Geometry check sheet. Reference: the model listing, model coordinates, mm. Coordinates: 2 decimals unless noted, no trailing zeros. Write each loop counter-clockwise with the first axis right and the second up, starting at its lowest first coordinate (ties: lowest second). Pieces come first, ordered by that corner, then holes. Notation, with made-up numbers: M 70.5,-33.5 L 120.5,-33.5 A23 cw 120.5,2.5 Z; hole C -8,40.25 d1. An arc over 180 degrees is marked long. Write item = value, one per line. Start each with the question number.
```python
from build123d import *

# Parameters (mm, degrees)
SKETCH5_W           = 40
SKETCH5_H           = 40
BOSS_EXTRUDE2_DEPTH = 2
CUT_EXTRUDE1_DEPTH  = 2
CUT_EXTRUDE4_DEPTH  = 2
CUT_EXTRUDE5_DEPTH  = 2
CUT_EXTRUDE6_DEPTH  = 2
CUT_EXTRUDE7_DEPTH  = 2
CUT_EXTRUDE8_DEPTH  = 2


with BuildPart() as part:
    # Sketch5 → Boss-Extrude2 (new body)
    with BuildSketch(Plane.XY):
        Rectangle(SKETCH5_W, SKETCH5_H)
    extrude(amount=BOSS_EXTRUDE2_DEPTH)

    # Sketch4 → Cut-Extrude1 (cut)
    with BuildSketch(Plane.XY):
        Polygon((18, 16.585786438), (18, 10.414213562), (14.914213562, 13.5), align=None)
        Polygon((10.414213562, 18.056847711), (16.585786438, 18.056847711), (13.5, 14.971061274), align=None)
    extrude(amount=CUT_EXTRUDE1_DEPTH, mode=Mode.SUBTRACT)

    # Sketch4_5 → Cut-Extrude4 (cut)
    with BuildSketch(Plane.XY):
        Polygon((-13.5, -14.914213562), (-16.585786438, -18), (-10.414213562, -18), align=None)
        Polygon((-5.914213562, -13.5), (-9, -16.585786438), (-12.085786438, -13.5), (-9, -10.414213562), align=None)
        Polygon((-13.5, -5.914213562), (-10.414213562, -9), (-13.5, -12.085786438), (-16.585786438, -9), align=None)
        Polygon((-18, -16.585786438), (-18, -10.414213562), (-14.914213562, -13.5), align=None)
    extrude(amount=CUT_EXTRUDE4_DEPTH, mode=Mode.SUBTRACT)

    # Sketch4_6 → Cut-Extrude5 (cut)
    with BuildSketch(Plane.XY):
        Polygon((-1.414213562, -18), (-7.585786438, -18), (-4.5, -14.914213562), align=None)
        Polygon((3.085786438, -13.5), (0, -16.585786438), (-3.085786438, -13.5), (0, -10.414213562), align=None)
        Polygon((7.585786438, -18), (1.414213562, -18), (4.5, -14.914213562), align=None)
        Polygon((12.085786438, -13.5), (9, -16.585786438), (5.914213562, -13.5), (9, -10.414213562), align=None)
        Polygon((13.5, -14.914213562), (16.585786438, -18), (10.414213562, -18), align=None)
        Polygon((18, -10.414213562), (18, -16.585786438), (14.914213562, -13.5), align=None)
        Polygon((13.5, -5.914213562), (16.585786438, -9), (13.5, -12.085786438), (10.414213562, -9), align=None)
        Polygon((4.5, -5.914213562), (7.585786438, -9), (4.5, -12.085786438), (1.414213562, -9), align=None)
        Polygon((12.085786438, -4.5), (9, -7.585786438), (5.914213562, -4.5), (9, -1.414213562), align=None)
        Polygon((18, -1.414213562), (18, -7.585786438), (14.914213562, -4.5), align=None)
    extrude(amount=CUT_EXTRUDE5_DEPTH, mode=Mode.SUBTRACT)

    # Sketch4_7 → Cut-Extrude6 (cut)
    with BuildSketch(Plane.XY):
        Polygon((13.5, 3.085786438), (16.585786438, 0), (13.5, -3.085786438), (10.414213562, 0), align=None)
        Polygon((18, 7.585786438), (18, 1.414213562), (14.914213562, 4.5), align=None)
        Polygon((13.5, 12.085786438), (16.585786438, 9), (13.5, 5.914213562), (10.414213562, 9), align=None)
        Polygon((12.085786438, 4.5), (9, 1.414213562), (5.914213562, 4.5), (9, 7.585786438), align=None)
        Polygon((4.5, 12.085786438), (7.585786438, 9), (4.5, 5.914213562), (1.414213562, 9), align=None)
        Polygon((12.085786438, 13.5), (9, 10.414213562), (5.914213562, 13.5), (9, 16.585786438), align=None)
        Polygon((1.357365851, 18.056847711), (7.642634149, 18.056847711), (4.5, 14.914213562), align=None)
        Polygon((3.085786438, 13.5), (0, 10.414213562), (-3.085786438, 13.5), (0, 16.585786438), align=None)
        Polygon((3.085786438, 4.5), (0, 1.414213562), (-3.085786438, 4.5), (0, 7.585786438), align=None)
        Polygon((4.5, 3.085786438), (7.585786438, 0), (4.5, -3.085786438), (1.414213562, 0), align=None)
        Polygon((3.085786438, -4.5), (0, -7.585786438), (-3.085786438, -4.5), (0, -1.414213562), align=None)
        Polygon((-4.5, -5.914213562), (-1.414213562, -9), (-4.5, -12.085786438), (-7.585786438, -9), align=None)
    extrude(amount=CUT_EXTRUDE6_DEPTH, mode=Mode.SUBTRACT)

    # Sketch4_9 → Cut-Extrude7 (cut)
    with BuildSketch(Plane.XY):
        Polygon((-9, 1.414213562), (-12.085786438, 4.5), (-9, 7.585786438), (-5.914213562, 4.5), align=None)
        Polygon((-4.5, 3.085786438), (-1.414213562, 0), (-4.5, -3.085786438), (-7.585786438, 0), align=None)
        Polygon((-9, -7.585786438), (-12.085786438, -4.5), (-9, -1.414213562), (-5.914213562, -4.5), align=None)
        Polygon((-13.5, 3.085786438), (-10.414213562, 0), (-13.5, -3.085786438), (-16.585786438, 0), align=None)
        Polygon((-18, -7.585786438), (-18, -1.414213562), (-14.914213562, -4.5), align=None)
        Polygon((-18, 1.414213562), (-18, 7.585786438), (-14.914213562, 4.5), align=None)
    extrude(amount=CUT_EXTRUDE7_DEPTH, mode=Mode.SUBTRACT)

    # Sketch4_10 → Cut-Extrude8 (cut)
    with BuildSketch(Plane.XY):
        Polygon((-4.5, 12.085786438), (-1.414213562, 9), (-4.5, 5.914213562), (-7.585786438, 9), align=None)
        Polygon((-9, 10.414213562), (-12.085786438, 13.5), (-9, 16.585786438), (-5.914213562, 13.5), align=None)
        Polygon((-13.5, 12.085786438), (-10.414213562, 9), (-13.5, 5.914213562), (-16.585786438, 9), align=None)
        Polygon((-14.914213562, 13.5), (-18, 10.414213562), (-18, 16.585786438), align=None)
        Polygon((-10.357365851, 18.056847711), (-13.5, 14.914213562), (-16.642634149, 18.056847711), align=None)
        Polygon((-7.642634149, 18.056847711), (-1.357365851, 18.056847711), (-4.5, 14.914213562), align=None)
    extrude(amount=CUT_EXTRUDE8_DEPTH, mode=Mode.SUBTRACT)


solid = part.part
```
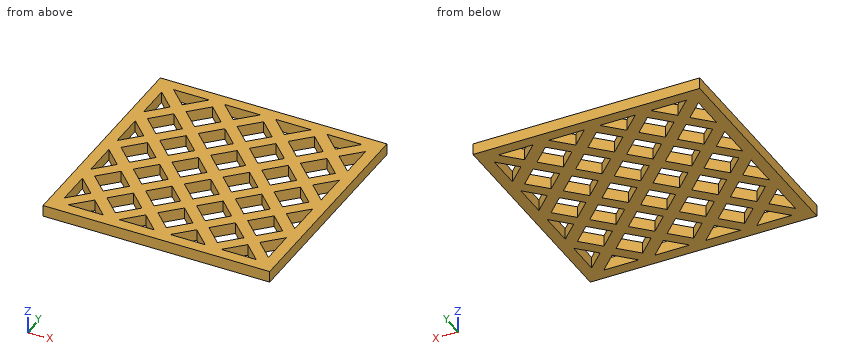
Q1. Cross-section at C-C on z = 1.65. Count the separate pieces of the cut face and the enclosed holes in it, and give its area (3 significant figures).
Q2. Cross-section at A-A on y = -4. Enter the section's corners in (x, z), and give its area (3 significant figures).
Q3. Gauge pin test, flat end, axial feed: pin 1 (12 mm diameter, centred on x = 13, y = 7, fed in from -Z). Record the tip position at first contact, or that the pin passes through.
Q4. Scan lines: L1, parallel to Y at x = 5, z = 1.3; L2, parallel to X at y = 8.5, z = 0.3; L3, parallel to Y at x = -5.5, z = 0.75. Record each from-to range of solid material in increasing order.
Q5. Cross-section at B-B on y = 17.5. Enter the section's corners in (x, z).
Values found:
q1.separate_pieces = 1
q1.enclosed_holes = 40
q1.area = 990 mm²
q2.outline = M -20,0 L -18,0 L -18,2 L -20,2 Z; M -15.41,0 L -11.59,0 L -11.59,2 L -15.41,2 Z; M -6.41,0 L -2.59,0 L -2.59,2 L -6.41,2 Z; M 2.59,0 L 6.41,0 L 6.41,2 L 2.59,2 Z; M 11.59,0 L 15.41,0 L 15.41,2 L 11.59,2 Z; M 18,0 L 20,0 L 20,2 L 18,2 Z
q2.area = 38.6 mm²
q3.pin_1 = 0
q4.L1 = -20 to -18, -15.41 to -11.59, -6.41 to -2.59, 2.59 to 6.41, 11.59 to 15.41, 18.06 to 20
q4.L2 = -20 to -16.09, -10.91 to -7.09, -1.91 to 1.91, 7.09 to 10.91, 16.09 to 20
q4.L3 = -20 to -18, -15.91 to -11.09, -6.91 to -2.09, 2.09 to 6.91, 11.09 to 15.91, 18.06 to 20
q5.outline = M -20,0 L -16.09,0 L -16.09,2 L -20,2 Z; M -10.91,0 L -7.09,0 L -7.09,2 L -10.91,2 Z; M -1.91,0 L 1.91,0 L 1.91,2 L -1.91,2 Z; M 7.09,0 L 10.97,0 L 10.97,2 L 7.09,2 Z; M 16.03,0 L 20,0 L 20,2 L 16.03,2 Z
